```python
from build123d import *

# Parameters (mm, degrees)
BOSS_EXTRUDE1_DEPTH = 52.5
FILLET1_R           = 7


with BuildPart() as part:
    # Sketch1 → Boss-Extrude1 (new, symmetric)
    with BuildSketch(Plane(origin=(0, 0, 0), x_dir=(0, 0, -1), z_dir=(1, 0, 0))):
        Polygon((-15.630670187, -4.507264222), (-15.630670187, 25.492735778), (9.369329813, 25.492735778), (9.369329813, -4.507264222), (6.093628879, -4.507264222), (6.093628879, 19.604885311), (-12.130670187, 19.604885311), (-12.130670187, -4.507264222), align=None)
    extrude(amount=BOSS_EXTRUDE1_DEPTH, both=True)

    # Fillet1
    fillet1_edges = [part.edges().sort_by_distance(p)[0] for p in [
        (0, 25.492735778, 15.630670187),
        (0, 25.492735778, -9.369329813),
    ]]
    fillet(fillet1_edges, radius=FILLET1_R)


solid = part.part
```
The listing builds one solid part. Answer for the finished solid, in the listing's coordinates (mm). A direction names the side the tool comes from. Coordinates: 2 decimals unless noted, no trailing zeros. Write each loop counter-clockwise with the first axis right and the second up, starting at its lowest first coordinate (ties: lowest second). Pieces come first, ordered by that corner, then holes. Notation, with made-up numbers: (10.25, -14) -> (47.25, -14) arc R23 cw to (47.25, 3) -> close; hole circle Ø8 at (19.5, -3.5). An arc over 180 degrees is marked (long way). Write each question's results on one line, items separated by ' | '. Start each with the question number.
1) For a pull along Z with two mould halves and no side action, classify faces 3 (the flat face through (1, 8, 12.131)), 4 (the flat face through (-52.5, 21, 3)), 5 (the flat face through (1, 7, 15.631)) as +Z half, -Z half, draft (parallel to the pull), parting line (faces both ways), or undercut.
2) A tool of negligible diameter and unlimited length cuts with its end or side. For faces 1 (the flat face through (52.5, 21, 3)), 2 (the flat face through (1, 7, -6.094)), from which of +Z, -Z, +X, -X, +Y, -Y can it reach the whole face along a straight path? Write none if from no direction.
3) A cutting plane is placed at C-C (z = 0.75). Determine the outline of the cut face in (x, y).
4) A cutting plane is placed at D-D (z = -4). Determine the outline of the cut face in (x, y), then the cut area to 3 significant figures.
5) A cutting plane is placed at B-B (x = -12). Determine the outline of the cut face in (y, z), then the cut area to 3 significant figures.
6) Flat-ended cylindrical pins translate along their axes: pin 1 Ø10 at (y, z) = (0.5, 1.5) entering from -X; pin 2 Ø5 at (x, z) = (17, 2.5) entering from -Y. Find the tip coordinate at first contact, or state that the pin passes through.
7) Straight lines are drawn through the part: probe 1 along Z at (x, y) = (25, 4); probe 2 along Y at (x, z) = (-16.5, 5.5); probe 3 along Y at (x, z) = (-5.5, -6.75). For each, find the intervals that lie inside material, in ascending order.
8) A cutting plane is placed at A-A (y = 16.5). Determine the outline of the cut face in (x, z), then the cut area to 3 significant figures.
Values follow:
1) face 3: undercut | face 4: draft | face 5: +Z half
2) face 1: +Z, -Z, +X, +Y, -Y | face 2: +X, -X, -Y
3) outline: (-52.5, 19.6) -> (52.5, 19.6) -> (52.5, 25.49) -> (-52.5, 25.49) -> close
4) outline: (-52.5, 19.6) -> (52.5, 19.6) -> (52.5, 25.3) -> (-52.5, 25.3) -> close | area: 598 mm²
5) outline: (-4.51, -9.37) -> (18.49, -9.37) arc R7 ccw to (25.49, -2.37) -> (25.49, 8.63) arc R7 ccw to (18.49, 15.63) -> (-4.51, 15.63) -> (-4.51, 12.13) -> (19.6, 12.13) -> (19.6, -6.09) -> (-4.51, -6.09) -> close | area: 290 mm²
6) pin 1: through | pin 2: y = 19.6
7) probe 1: -9.37 to -6.09, 12.13 to 15.63 | probe 2: 19.6 to 25.49 | probe 3: -4.51 to 23.95
8) outline: (-52.5, -9.37) -> (52.5, -9.37) -> (52.5, -6.09) -> (-52.5, -6.09) -> close; (-52.5, 12.13) -> (52.5, 12.13) -> (52.5, 15.63) -> (-52.5, 15.63) -> close | area: 711 mm²
